```python
from build123d import *

# Parameters (mm, degrees)
F0_R     = 350
F0_W     = 60.5
F0_H     = 25.5
F1_DEPTH = 5
F2_DEPTH = 2
F3_R     = 5
F4_DEPTH = 1


with BuildPart() as f1:
    # F0 (on Top) → F1 (new body)
    with BuildSketch(Plane.XY):
        Circle(F0_R)
        Rectangle(F0_W, F0_H, mode=Mode.SUBTRACT)
        Rectangle(F0_W, F0_H)
    extrude(amount=-F1_DEPTH)

    # F0 (on Top) → F2 (cut)
    with BuildSketch(Plane.XY):
        Rectangle(F0_W, F0_H)
    extrude(amount=-F2_DEPTH, mode=Mode.SUBTRACT)

    # F3 (on face) → F4 (cut)
    with BuildSketch(Plane.XY.offset(-2)):
        Circle(F3_R)
    extrude(amount=-F4_DEPTH, mode=Mode.SUBTRACT)


solid = f1.part
```
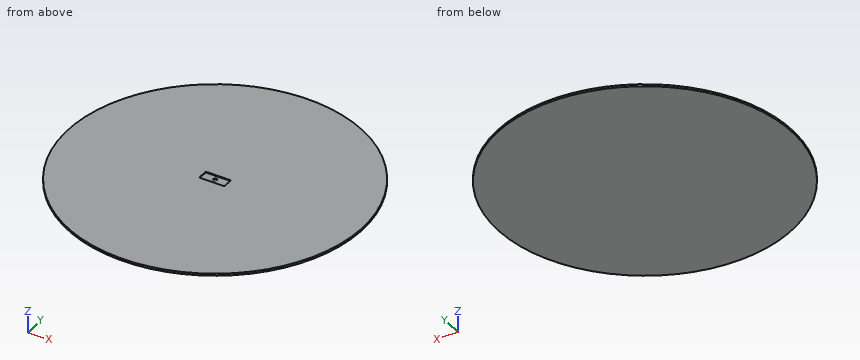
The model under review builds one solid part; all positions refer to its coordinate system, in mm. Give positions to 0.01 mm unless a question says otherwise; leave off trailing zeros. Write each loop counter-clockwise with the first axis right and the second up, starting at its lowest first coordinate (ties: lowest second). Pieces come first, ordered by that corner, then holes. Notation, with made-up numbers: (37.5, -14) -> (43.5, -14) arc R28 ccw to (43.5, 17) -> close; hole circle Ø8 at (-24, -6). An arc over 180 degrees is marked (long way). Answer in a Markdown table with one row per item.
1) Add section A-A on z = -4.2. State the section outline as (x, y) points.
Worked answers:
| item | result |
|---|---|
| outline | circle Ø700 at (0, 0) |
2) Add section B-B on x = 130. State the section outline as (y, z) points.
Worked answers:
| item | result |
|---|---|
| outline | (-324.96, -5) -> (324.96, -5) -> (324.96, 0) -> (-324.96, 0) -> close |
3) Add section C-C on y = 68.5. State the section outline as (x, z) points.
Worked answers:
| item | result |
|---|---|
| outline | (-343.23, -5) -> (343.23, -5) -> (343.23, 0) -> (-343.23, 0) -> close |
4) For L1, parallel to Y at x = 0, z = -2.45; L2, parallel to Y at x = -22.5, z = -0.25; L3, parallel to Y at x = 313, z = -2.9, list the stretches that pass through material, from the lowest coordinate up. Write a range as [from, to].
Worked answers:
| item | result |
|---|---|
| L1 | [-350, -5], [5, 350] |
| L2 | [-349.28, -12.75], [12.75, 349.28] |
| L3 | [-156.62, 156.62] |
5) Clearance check with flat-ended pins moving along their axes: P1, Ø11.5, axis at x = 0, y = 0, coming from the +Z side; P2, Ø1.5, axis at y = -32, z = -1.5, coming from the -X side; P3, Ø1.5, axis at y = 123, z = -3.5, coming from the -X side. State where each tip first meets the part, or that it passes through.
Worked answers:
| item | result |
|---|---|
| P1 | z = -2 |
| P2 | x = -348.6 |
| P3 | x = -327.96 |
